```python
from build123d import *

# Parameters (mm, degrees)
SKETCH1_R           = 304.8
BOSS_EXTRUDE1_DEPTH = 914.4
SKETCH2_OUTSIDE_W   = 862.944
SKETCH2_OUTSIDE_H   = 862.944
SKETCH2_OUTSIDE_R   = 304.8
SKETCH2_OUTSIDE_R_2 = 279.4
CUT_EXTRUDE2_DEPTH  = 889
SKETCH3_R           = 12.7
CUT_EXTRUDE3_DEPTH  = 25.4


with BuildPart() as part:
    # Sketch1 → Boss-Extrude1 (new body)
    with BuildSketch(Plane(origin=(0, 0, 0), x_dir=(1, 0, 0), z_dir=(0, 1, 0))):
        Circle(SKETCH1_R)
    extrude(amount=BOSS_EXTRUDE1_DEPTH)

    # Sketch2 outside → Cut-Extrude2 (cut)
    with BuildSketch(Plane(origin=(0, 914.4, 0), x_dir=(1, 0, 0), z_dir=(0, 1, 0))):
        Rectangle(SKETCH2_OUTSIDE_W, SKETCH2_OUTSIDE_H)
        Circle(SKETCH2_OUTSIDE_R, mode=Mode.SUBTRACT)
        Circle(SKETCH2_OUTSIDE_R_2)
    extrude(amount=-CUT_EXTRUDE2_DEPTH, mode=Mode.SUBTRACT)

    # Sketch3 → Cut-Extrude3 (cut)
    with BuildSketch(Plane.XZ):
        Circle(SKETCH3_R)
    extrude(amount=-CUT_EXTRUDE3_DEPTH, mode=Mode.SUBTRACT)


solid = part.part
```
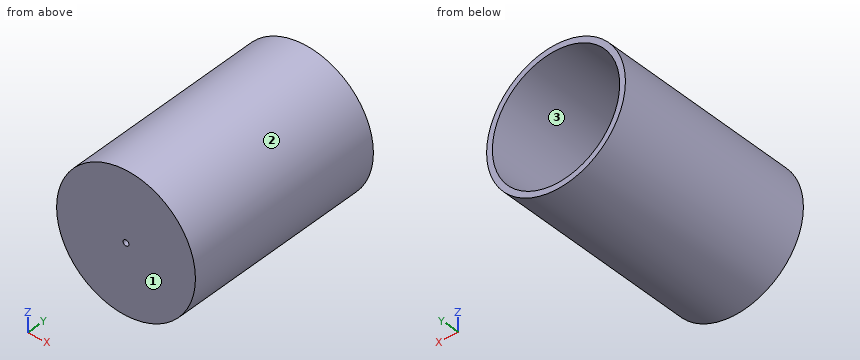
Read the model definition and answer for the solid it produces. Units are mm, in the model's axes. Face numbers are marked on the shaded views. Round coordinates to 2 decimals unless told otherwise and drop trailing zeros. Write each loop counter-clockwise with the first axis right and the second up, starting at its lowest first coordinate (ties: lowest second). Pieces come first, ordered by that corner, then holes. Notation, with made-up numbers: (-32.5, -12.75) -> (-28.5, -12.75) arc R22 ccw to (-28.5, 25.25) -> close; hole circle Ø6 at (33, 15). An arc over 180 degrees is marked (long way). Answer in a Markdown table with one row per item. Add a question column.
1) Find section B-B, the plane x = 0. Determine the outline of the cut face in (y, z), and give its area (3 significant figures).
2) Find section A-A, the plane z = 0. Determine the outline of the cut face in (x, y), and give its area (3 significant figures).
3) Determine the mould class of the marked faces 1, 2 and 3 for opening direction Z: pulls with the +Z half, pulls with the -Z half, needs draft (parallel to the pull), parting line crosses it, or undercut.
4) Consider line 1 (X direction, y = 573, z = 0); line 2 (Z direction, x = 0, y = 8.5). Determine where each line is inside the solid, lowest interval first.
5) Find section C-C, the plane z = 228. Determine the outline of the cut face in (x, y), and give its area (3 significant figures).
6) Find section D-D, the plane y = 416. Determine the outline of the cut face in (x, z).
7) Given P1, Ø10, axis at x = -150.5, z = -42.5, coming from the +Y side; P2, Ø8, axis at x = 19, y = 466.5, coming from the -Z side; P3, Ø8, axis at y = 261.5, z = -56.5, coming from the -X side, each flat-ended and moving along its own axis, determine where each tip first touches the part or whether it passes through.
Findings below:
| question | item | result |
|---|---|---|
| 1 | outline | (0, -304.8) -> (914.4, -304.8) -> (914.4, -279.4) -> (25.4, -279.4) -> (25.4, -12.7) -> (0, -12.7) -> close; (0, 12.7) -> (25.4, 12.7) -> (25.4, 279.4) -> (914.4, 279.4) -> (914.4, 304.8) -> (0, 304.8) -> close |
| 1 | area | 60,000 mm² |
| 2 | outline | (-304.8, 0) -> (-12.7, 0) -> (-12.7, 25.4) -> (-279.4, 25.4) -> (-279.4, 914.4) -> (-304.8, 914.4) -> close; (12.7, 0) -> (304.8, 0) -> (304.8, 914.4) -> (279.4, 914.4) -> (279.4, 25.4) -> (12.7, 25.4) -> close |
| 2 | area | 60,000 mm² |
| 3 | face 1 | needs draft |
| 3 | face 2 | parting line crosses it |
| 3 | face 3 | undercut |
| 4 | line 1 | -304.8 to -279.4, 279.4 to 304.8 |
| 4 | line 2 | -304.8 to -12.7, 12.7 to 304.8 |
| 5 | outline | (-202.28, 0) -> (202.28, 0) -> (202.28, 914.4) -> (161.49, 914.4) -> (161.49, 25.4) -> (-161.49, 25.4) -> (-161.49, 914.4) -> (-202.28, 914.4) -> close |
| 5 | area | 82,800 mm² |
| 6 | outline | circle Ø609.6 at (0, 0); hole circle Ø558.8 at (0, 0) |
| 7 | P1 | y = 25.4 |
| 7 | P2 | z = -304.43 |
| 7 | P3 | x = -300.24 |
